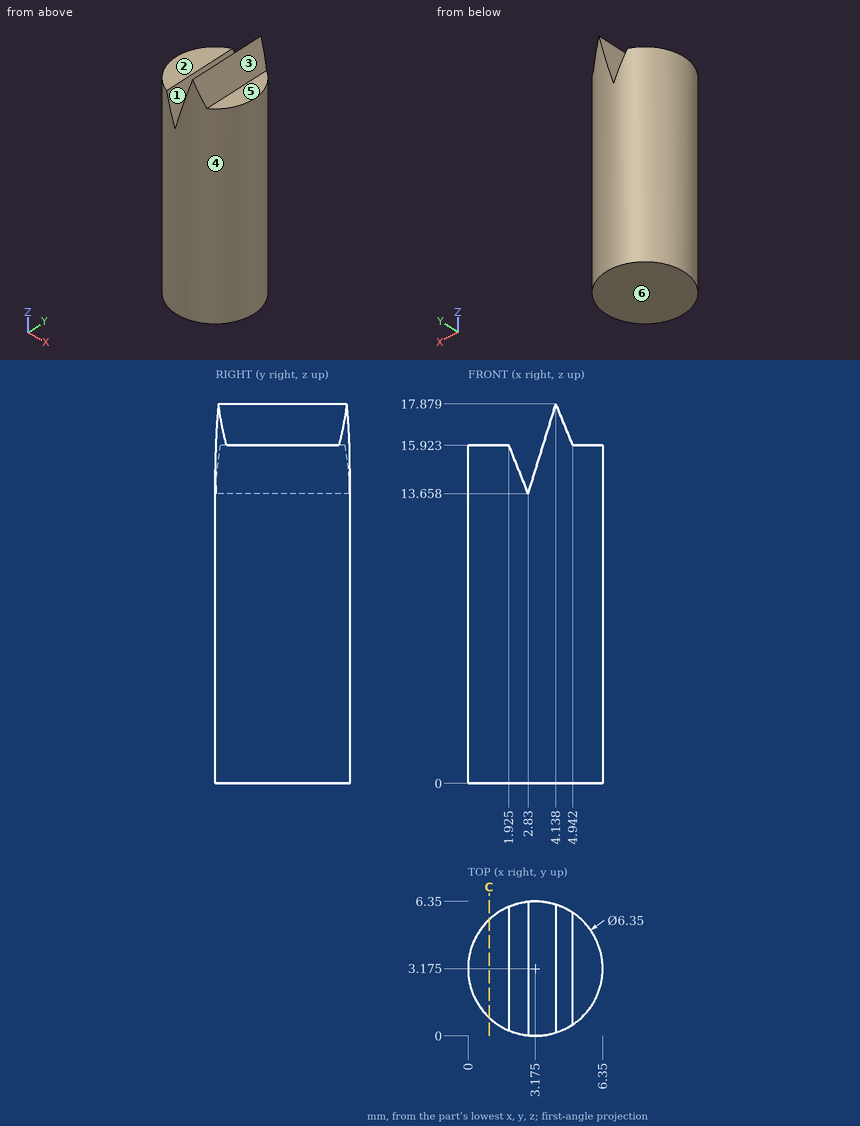
For this review, use the dimensioned drawing (mm, ordinates from the lowest corner) and the shaded views. A direction names the side the tool comes from. Round coordinates to 2 decimals unless told otherwise and drop trailing zeros. Order: outer loops, then holes, each group sorted by start corner. A loop starts at its lowest first (then second) coordinate and runs counter-clockwise, first axis right, second up. Notation, with made-up numbers: (27, 88.5) -> (70, 88.5) arc R8 cw to (70, 95.5) -> close; hole circle Ø8 at (15, 27). An arc over 180 degrees is marked (long way). Write item = value, one per line. Start each with the question number.
Item 1: Mouldability with a two-part tool opening along X and no side actions: class the marked faces 1, 2, 3 and 4 as released by +X, released by -X, zero draft, split by the parting line, or undercut.
Item 2: Consider section C-C on x = 1. Write out the cut boundary in (y, z).
Item 3: For line 1 along Z through (x, y) = (1.75, 2.5); line 2 along X through (y, z) = (2.25, 15) (1 decimal); line 3 along X through (y, z) = (5.25, 14.25) (1 decimal), list the stretches that pass through material, from the lowest coordinate up.
Item 4: For the marked faces 5 and 6, list the 3-axis set-ups (+Z, -Z, +X, -X, +Y, -Y) from which the entire face can be reached by the end or side of a thin tool; tool diameter is ignored.
Item 5: Clearance check with flat-ended pins moving along their axes: pin 1 Ø3 at (y, z) = (2.5, 7) entering from +X; pin 2 Ø0.6 at (x, y) = (1, 4.5) entering from +Z; pin 3 Ø1 at (y, z) = (0.5, 12) entering from +X; pin 4 Ø1.5 at (y, z) = (5, 10.5) entering from +X. State where each tip first meets the part, or that it passes through.
Conclusion:
q1.face_1 = undercut
q1.face_2 = zero draft
q1.face_3 = released by +X
q1.face_4 = split by the parting line
q2.outline = (0.86, 0) -> (5.49, 0) -> (5.49, 15.92) -> (0.86, 15.92) -> close
q3.line_1 = 0 to 15.92
q3.line_2 = 0.1 to 2.3, 3.2 to 6.2
q3.line_3 = 0.8 to 2.6, 3 to 5.6
q4.face_5 = +Z, +X, +Y, -Y
q4.face_6 = -Z, +X, -X, +Y, -Y
q5.pin_1 = 6.35
q5.pin_2 = 15.92
q5.pin_3 = 5.49
q5.pin_4 = 6.16
